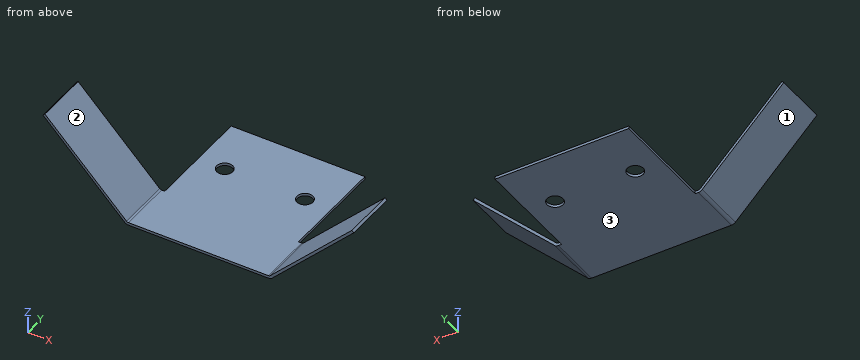
Autodesk Inventor part; units mm, degrees
ref_plane "YZ Plane" through (0, 0, 0) normal (1, 0, 0) x (0, 1, 0)
ref_plane "XZ Plane" through (0, 0, 0) normal (0, 1, 0) x (-1, 0, 0)
ref_plane "XY Plane" through (0, 0, 0) normal (0, 0, 1) x (1, 0, 0)
sketch "Sketch1" plane through (0, 0, 0) normal (0, 0, 1) x (1, 0, 0)
  line L0 (0, 0) -> (0, 10)
  line L1 (0, 10) -> (21, 10)
  line L2 (22, 10) -> (22, 30)
  line L3 (22, 30) -> (47, 30)
  line L4 (47, 30) -> (47, 10)
  line L5 (48, 10) -> (69, 10)
  line L6 (69, 10) -> (69, 0)
  line L7 (21, 10) -> (21, 0)
  line L8 (48, 10) -> (48, 0)
  line L9 (69, 0) -> (48, 0)
  line L10 (21, 0) -> (0, 0)
  line L11 (21, 0) -> (48, 0)
  line L12 (48, 10) -> (47, 10)
  line L13 (21, 10) -> (22, 10)
  dimension "d0" = 22
  dimension "d1" = 22
  dimension "d2" = 10
  dimension "d3" = 25
  dimension "d5" = 10
  dimension "d8" = 1
  dimension "d9" = 1
extrude "Plate1" add sketch "Sketch1" along normal blind 0.5 contours L7 L13 L2 L3 L4 L12 L8 L11
sketch "Sketch2" plane through (21.3536, 0, 0.3536) normal (-0.7071068, 0, -0.7071068) x (0, -1, 0)
  line L0 (-10, 0) -> (0, 0)
  line L1 (0, 0) -> (0, 22)
  line L2 (0, 22) -> (-10, 22)
  line L3 (-10, 22) -> (-10, 0)
edge flange "Flange1" height 22 angle 45 thickness 0.5 bend radius 0.5 thickness toward (-0.7071068, 0, -0.7071068) relief straight relief width 0.5 relief depth 0.25 corner gap 0.5 corner form 0 edges at (21, 5, 0.5) (48, 5, 0.5) wall of the first edge with corners at (21.3536, 10, 0.3536) (21.3536, 0, 0.3536) (5.7972, 0, 15.9099) (5.7972, 10, 15.9099)
bend "Bend1"
corner "Corner1"
sketch "Sketch3" plane through (0, 0, 0) normal (0, 0, -1) x (-1, 0, 0)
  line L0 (-21.4142, 0) -> (-47.5858, 0)
  line L1 (-47, 10) -> (-47, 30)
  circle A0 centre (-42, 20) radius 1.5
  circle A1 centre (-27, 20) radius 1.5
  point P0 (0, 0)
  dimension "d21" = 3
  dimension "d22" = 3
  dimension "d23" = 15
  dimension "d24" = 20
  dimension "d25" = 5
hole "Hole1" at (42, 20, 0) at (27, 20, 0) direction (0, 0, 1) diameter 3 depth 0.5 tip angle 118
equation "\"d31\" = Thickness"
equation "\"d11\" = BendReliefWidth"
equation "\"d12\" = BendReliefDepth"
equation "\"d13\" = MinimumRemnant"
equation "\"d14\" = BendRadius"
equation "\"d17\" = BendRadius"
equation "\"d18\" = CornerReliefSize"
equation "\"d19\" = GapSize"
equation "\"d20\" = JacobiRadiusSize"
equation "\"BendRadius\" = Thickness"
equation "\"BendReliefWidth\" = Thickness"
equation "\"BendReliefDepth\" = 0.5 * Thickness"
equation "\"CornerReliefSize\" = 4 * Thickness"
equation "\"MinimumRemnant\" = 2 * Thickness"
equation "\"TransitionRadius\" = BendRadius"
equation "\"JacobiRadiusSize\" = Thickness"
equation "\"GapSize\" = Thickness"
equation "\"d10\" = BendRadius"
properties part number "PÁRA LAMA TRASEIRO"
Build history of the part. All positions in model axes, mm. Face numbers are marked on the shaded views. Coordinates: 2 decimals unless noted, no trailing zeros. Write each loop counter-clockwise with the first axis right and the second up, starting at its lowest first coordinate (ties: lowest second). Pieces come first, ordered by that corner, then holes.
1. Band-saw the part on C-C, the plane z = 6.75. Give the cut face in (x, y).
Answer block:
outline: (14.25, 0) - (14.96, 0) - (14.96, 10) - (14.25, 10) - close; (54.04, 0) - (54.75, 0) - (54.75, 10) - (54.04, 10) - close
2. Pull direction X, two halves, no side cores. Call the marked faces 1, 2 and 3: released by +X, released by -X, zero draft, split by the parting line, or undercut.
Answer block:
face 1: released by -X
face 2: undercut
face 3: zero draft
3. Drop flat-ended pins along their axis: pin 1 (8 mm diameter, centred on x = 34, y = 21.5, fed in from +Z); pin 2 (4 mm diameter, centred on y = 9.5, z = 2, fed in from +X); pin 3 (1 mm diameter, centred on x = 54, y = 10, fed in from +Z); pin 4 (2.5 mm diameter, centred on x = 27, y = 20, fed in from +Z). Give the stop position or say it passes through.
Answer block:
pin 1: stops at z = 0.5
pin 2: stops at x = 52
pin 3: stops at z = 7.21
pin 4: passes through
4. Band-saw the part on D-D, the plane y = 5.75. Give the cut face in (x, z), and give its area (3 significant figures).
Answer block:
outline: (5.44, 15.56) - (20.71, 0.29) arc R1 ccw to (21.41, 0) - (47.59, 0) arc R1 ccw to (48.29, 0.29) - (63.56, 15.56) - (63.2, 15.91) - (47.94, 0.65) arc R0.5 cw to (47.59, 0.5) - (21.41, 0.5) arc R0.5 cw to (21.06, 0.65) - (5.8, 15.91) - close
area: 35.3 mm2
5. Band-saw the part on B-B, the plane y = 20. Give the cut face in (x, z), and give its area (3 significant figures).
Answer block:
outline: (22, 0) - (25.5, 0) - (25.5, 0.5) - (22, 0.5) - close; (28.5, 0) - (40.5, 0) - (40.5, 0.5) - (28.5, 0.5) - close; (43.5, 0) - (47, 0) - (47, 0.5) - (43.5, 0.5) - close
area: 9.50 mm2
6. Drill centre lines: probe 1 along X at (y, z) = (20, 0.3); probe 2 along Y at (x, z) = (27, 0.45); probe 3 along Z at (x, y) = (27, 2.5). Where is each one in solid material? Low to high.
Answer block:
probe 1: x = 22 to 25.5, 28.5 to 40.5, 43.5 to 47
probe 2: y = 0 to 18.5, 21.5 to 30
probe 3: z = 0 to 0.5
7. Band-saw the part on A-A, the plane x = 42. Give the cut face in (y, z), and give its area (3 significant figures).
Answer block:
outline: (0, 0) - (18.5, 0) - (18.5, 0.5) - (0, 0.5) - close; (21.5, 0) - (30, 0) - (30, 0.5) - (21.5, 0.5) - close
area: 13.5 mm2
